Design review of the part built by this model. Coordinates are the model's own, in mm. A direction names the side the tool comes from. Coordinates: 2 decimals unless noted, no trailing zeros. Loops run counter-clockwise (first coordinate to the right, second up) from the corner with the lowest first, then second, coordinate; pieces in that order, holes last. Notation, with made-up numbers: (44.5, 36.5) - (60.5, 36.5) arc R26 cw to (60.5, 61.5) - close; hole circle Ø10 at (57.25, 68). An arc over 180 degrees is marked (long way). Use one line per item in the form item = value. Start each with the question number.
(1) Add section B-B (y = 54). State the section outline as (x, z) points, plus the area to 3 significant figures.
(2) Tool access review of faces 4 (the face through (-26, 25.4, 25)), 5 (the face through (-31, 50.8, 35)), 6 (the face through (0, 7.62, 25)), 7 (the face through (-43, 49, 17.78)): name each direction out of +Z, -Z, +X, -X, +Y, -Y from which nothing blocks a thin tool from reaching the whole face with its end or side.
(3) Add section A-A (z = 13.5). State the section outline as (x, y) points (1 decimal), plus the area to 3 significant figures.
(4) Clearance check with flat-ended pins moving along their axes: pin 1 Ø13 at (x, z) = (28.5, 40.5) entering from +Y; pin 2 Ø19 at (y, z) = (56, 42) entering from +X; pin 3 Ø12 at (y, z) = (47, 39) entering from -X; pin 4 Ø10 at (x, y) = (55, 12.5) entering from -Z. State where each tip first meets the part, or that it passes through.
(5) For L1, parallel to X at y = 17, z = 46.5; L2, parallel to Y at x = -56, z = 14.5; L3, parallel to X at y = 41, z = 22.5, list the stretches that pass through material, from the lowest coordinate up.
(6) Add section D-D (y = 45). State the section outline as (x, z) points, plus the area to 3 significant figures.
(7) The part is to be moulded in two halves that separate along X. For faces 1 (the face through (-11.853, 6, 25)), 2 (the face through (63.5, 24, 25)), 3 (the face through (51, 14, 40.64)), say which applies: pulls with the +X half, pulls with the -X half, needs draft (parallel to the pull), parting line crosses it, or undercut.
```python
from build123d import *

# Parameters (mm, degrees)
BOSS_EXTRUDE1_DEPTH = 50.8
BOSS_EXTRUDE2_DEPTH = 33.02
FILLET2_R           = 1.5875
CUT_EXTRUDE1_REACH  = 152.804
SKETCH3_W           = 30.48
SKETCH3_H           = 12.7


with BuildPart() as part:
    # Sketch1 → Boss-Extrude1 (new body)
    with BuildSketch(Plane.XY):
        Polygon((-63.5, 0), (-63.5, 38.1), (63.5, 38.1), (63.5, 0), (39.793333333, 0), (39.793333333, 25.4), (11.853333333, 25.4), (11.853333333, 0), (-11.853333333, 0), (-11.853333333, 25.4), (-39.793333333, 25.4), (-39.793333333, 0), align=None)
    extrude(amount=BOSS_EXTRUDE1_DEPTH)

    # Sketch2 → Boss-Extrude2 (add)
    with BuildSketch(Plane.XY.offset(50.8)):
        Polygon((55.876679783, 38.1), (55.876679783, 63.5), (40.636679783, 63.5), (40.636679783, 50.8), (22.856679783, 50.8), (22.856679783, 38.1), align=None)
    boss_extrude2 = extrude(amount=-BOSS_EXTRUDE2_DEPTH)

    # Mirror1: Boss-Extrude2 across plane
    add(boss_extrude2.mirror(Plane(origin=(0, 0, 0), x_dir=(0, 0, 1), z_dir=(1, 0, 0))))

    # Fillet2
    fillet2_edges = [part.edges().sort_by_distance(p)[0] for p in [
        (39.793333333, 25.4, 25.4),
        (11.853333333, 25.4, 25.4),
        (-11.853333333, 25.4, 25.4),
        (-39.793333333, 25.4, 25.4),
        (39.366679783, 38.1, 17.78),
        (55.876679783, 38.1, 34.29),
        (22.856679783, 38.1, 34.29),
        (40.636679783, 50.8, 34.29),
        (-22.856679783, 38.1, 34.29),
        (-55.876679783, 38.1, 34.29),
        (-40.636679783, 50.8, 34.29),
        (-39.366679783, 38.1, 17.78),
    ]]
    fillet(fillet2_edges, radius=FILLET2_R)

    # Cut-Extrude1: up to this face of the body (flat: up to its plane)
    cut_extrude1_end = Plane(part.part.faces().sort_by_distance((63.5, 19.05, 25.4))[0])
    # Sketch3 → Cut-Extrude1 (cut, up to the picked face)
    with BuildSketch(Plane.ZY.offset(63.5), mode=Mode.PRIVATE) as cut_extrude1_sk1:
        with Locations((25.4, 13.97)):
            Rectangle(SKETCH3_W, SKETCH3_H)
    cut_extrude1_tool1 = split(extrude(cut_extrude1_sk1.sketch, amount=-CUT_EXTRUDE1_REACH, mode=Mode.PRIVATE), bisect_by=cut_extrude1_end, keep=Keep.BOTH, mode=Mode.PRIVATE)
    add(cut_extrude1_tool1.solids().sort_by(Axis((-63.5, 13.97, 25.4), (1, 0, 0)))[0], mode=Mode.SUBTRACT)


solid = part.part
```
Computed values:
q1.outline = (-55.88, 17.78) - (-40.64, 17.78) - (-40.64, 50.8) - (-55.88, 50.8) - close; (40.64, 17.78) - (55.88, 17.78) - (55.88, 50.8) - (40.64, 50.8) - close
q1.area = 1,010 mm^2
q2.face_4 = +Z, -Z, -Y
q2.face_5 = +Z, -Z, +Y
q2.face_6 = +X, -X
q2.face_7 = -Z, +X, -X, +Y
q3.outline = (-63.5, 0) - (-39.8, 0) - (-39.8, 7.6) - (-63.5, 7.6) - close; (-63.5, 20.3) - (-39.8, 20.3) - (-39.8, 23.8) arc R1.6 cw to (-38.2, 25.4) - (-13.4, 25.4) arc R1.6 cw to (-11.9, 23.8) - (-11.9, 20.3) - (11.9, 20.3) - (11.9, 23.8) arc R1.6 cw to (13.4, 25.4) - (38.2, 25.4) arc R1.6 cw to (39.8, 23.8) - (39.8, 20.3) - (63.5, 20.3) - (63.5, 38.1) - (-63.5, 38.1) - close; (-11.9, 0) - (11.9, 0) - (11.9, 7.6) - (-11.9, 7.6) - close; (39.8, 0) - (63.5, 0) - (63.5, 7.6) - (39.8, 7.6) - close
q3.area = 2,520 mm^2
q4.pin_1 = 50.8
q4.pin_2 = 55.88
q4.pin_3 = -55.88
q4.pin_4 = 0
q5.L1 = -63.5 to -39.79, -11.85 to 11.85, 39.79 to 63.5
q5.L2 = 0 to 7.62, 20.32 to 38.1
q5.L3 = -55.88 to -22.86, 22.86 to 55.88
q6.outline = (-55.88, 17.78) - (-22.86, 17.78) - (-22.86, 50.8) - (-55.88, 50.8) - close; (22.86, 17.78) - (55.88, 17.78) - (55.88, 50.8) - (22.86, 50.8) - close
q6.area = 2,180 mm^2
q7.face_1 = undercut
q7.face_2 = pulls with the +X half
q7.face_3 = needs draft
